Part model, mm, in its own coordinate system. A direction names the side the tool comes from. Round coordinates to 2 decimals unless told otherwise and drop trailing zeros. Write each loop counter-clockwise with the first axis right and the second up, starting at its lowest first coordinate (ties: lowest second). Pieces come first, ordered by that corner, then holes.
from build123d import *

# Parameters (mm, degrees)
EXTRUDE_1_DEPTH      = 10
EXTRUDE_1_DEPTH_BACK = 48
SKETCH_2_R           = 8
SKETCH_3_W           = 4.4
SKETCH_3_H           = 8
EXTRUDE_2_DEPTH      = 14


with BuildPart() as part:
    # 草图1 → 旋转1 (revolve)
    with BuildSketch(Plane.XY, mode=Mode.PRIVATE) as revolve_1_sk:
        with BuildLine():
            Line((20, 0), (25, 0))
            Line((25, 0), (25, 24))
            Line((25, 24), (20, 32.660254038))
            Line((20, 32.660254038), (20, 50))
            ThreePointArc((20, 50), (10, 53.819660113), (0, 50))
            Line((0, 50), (0, 32.660254038))
            Line((0, 32.660254038), (-5, 24))
            Line((-5, 24), (-5, 12))
            Line((-5, 12), (-13, 12))
            Line((-13, 12), (-13, 0))
            Line((-13, 0), (-5, 0))
            Line((-5, 0), (0, 0))
            Line((0, 0), (20, 0))
        make_face()
    revolve(revolve_1_sk.sketch.rotate(Axis((0, 0, 0), (1, 0, 0)), 90), axis=Axis((0, 0, 0), (1, 0, 0)))

    # 草图2 → 凸台-拉伸1 (add, two sides: drawn at the far end of the back side and taken through both)
    with BuildSketch(Plane.ZY.offset(13).offset(-EXTRUDE_1_DEPTH_BACK)):
        Circle(SKETCH_2_R)
    extrude(amount=EXTRUDE_1_DEPTH + EXTRUDE_1_DEPTH_BACK)

    # 草图3 → 凸台-拉伸2 (add)
    with BuildSketch(Plane(origin=(0, 0, 0), x_dir=(1, 0, 0), z_dir=(0, 1, 0))):
        with Locations((-9, 0)):
            Rectangle(SKETCH_3_W, SKETCH_3_H)
    extrude(amount=EXTRUDE_2_DEPTH)


solid = part.part
Q1. Saw through at C-C, the plane x = 6. Write the cut outline in (y, z).
Q2. Saw through at B-B, the plane z = 0. Write the cut outline in (x, y), and give its area (3 significant figures).
Q3. Saw through at A-A, the plane y = 0. Write the cut outline in (x, z), and give its area (3 significant figures).
Q4. Saw through at D-D, the plane x = 17. Write the cut outline in (y, z), and give its area (3 significant figures).
Q5. Wall check: line 1 (X direction, y = 19.5, z = 3.5); line 2 (X direction, y = 47, z = -8); line 3 (Z direction, x = 14, y = 46.5). Give the ranges that are in metal, low to high.
Q6. Drop flat-ended pins along their axis: P1, Ø1.3, axis at x = -10, y = 12.5, coming from the -Z side; P2, Ø1.5, axis at x = -4.5, z = 14, coming from the -Y side; P3, Ø12, axis at x = -16, z = -6, coming from the +Y side. Give the stop position or say it passes through.
Q7. Tool access for faces 1 (the cylindrical face through (30.07, -7.81, -1.73)), 2 (the flat face through (-9, 14, 0)), 3 (the flat face through (0, 33, 10)), 4 (the flat face through (-9, 13, -4)): list every direction of +Z, -Z, +X, -X, +Y, -Y with a clear straight run to the whole face (end or side of a thin tool).
Computed:
1. outline: circle Ø106.55 at (0, 0)
2. outline: (-23, -8) - (-13, -8) - (-13, -12) - (-5, -12) - (-5, -24) - (0, -32.66) - (0, -50) arc R15 ccw to (20, -50) - (20, -32.66) - (25, -24) - (25, -8) - (35, -8) - (35, 8) - (25, 8) - (25, 24) - (20, 32.66) - (20, 50) arc R15 ccw to (0, 50) - (0, 32.66) - (-5, 24) - (-5, 12) - (-6.8, 12) - (-6.8, 14) - (-11.2, 14) - (-11.2, 12) - (-13, 12) - (-13, 8) - (-23, 8) - close
2. area: 3,190 mm2
3. outline: (-23, -8) - (-13, -8) - (-13, -12) - (-5, -12) - (-5, -24) - (0, -32.66) - (0, -50) arc R15 ccw to (20, -50) - (20, -32.66) - (25, -24) - (25, -8) - (35, -8) - (35, 8) - (25, 8) - (25, 24) - (20, 32.66) - (20, 50) arc R15 ccw to (0, 50) - (0, 32.66) - (-5, 24) - (-5, 12) - (-13, 12) - (-13, 8) - (-23, 8) - close
3. area: 3,180 mm2
4. outline: circle Ø104.17 at (0, 0)
4. area: 8,520 mm2
5. line 1: x = -5 to 25
5. line 2: x = 0 to 20
5. line 3: z = -26 to 26
6. P1: stops at z = -4
6. P2: stops at y = -22.18
6. P3: stops at y = 14
7. face 1: +X
7. face 2: +Z, -Z, -X, +Y
7. face 3: -X
7. face 4: -Z, -X, +Y
